Source: CAD feature listing. Evaluate the final solid. Frame: model axes, mm. Face numbers are marked on the shaded views. A direction names the side the tool comes from. Round coordinates to 2 decimals unless told otherwise and drop trailing zeros. Order: outer loops, then holes, each group sorted by start corner. A loop starts at its lowest first (then second) coordinate and runs counter-clockwise, first axis right, second up.
```python
from build123d import *

# Parameters (mm, degrees)
SKETCH1_W           = 6
SKETCH1_H           = 18
BOSS_EXTRUDE1_DEPTH = 2
SKETCH2_R           = 1.5
BOSS_EXTRUDE2_DEPTH = 3
FILLET1_R           = 1.5
SKETCH3_R           = 1.5
SKETCH5_R           = 1
CUT_EXTRUDE1_DEPTH  = 21.686831601


with BuildPart() as part:
    # Sketch1 → Boss-Extrude1 (new body)
    with BuildSketch(Plane.XY):
        Rectangle(SKETCH1_W, SKETCH1_H)
    extrude(amount=BOSS_EXTRUDE1_DEPTH)

    # Sketch2 → Boss-Extrude2 (add)
    with BuildSketch(Plane(origin=(0, 0, 0), x_dir=(-1, 0, 0), z_dir=(0, 0, -1))):
        with Locations((0, 2.35)):
            Circle(SKETCH2_R)
        with Locations((0, -2.62)):
            Circle(SKETCH2_R)
    extrude(amount=BOSS_EXTRUDE2_DEPTH)

    # Fillet1
    fillet1_edges = [part.edges().sort_by_distance(p)[0] for p in [
        (1.5, 2.35, -3),
        (1.5, -2.62, -3),
    ]]
    fillet(fillet1_edges, radius=FILLET1_R)

    # Sweep1: sweep along a path in Sketch4
    with BuildLine(Plane(origin=(0, 2.35, 0), x_dir=(-1, 0, 0), z_dir=(0, 1, 0))) as sweep1_path:
        Line((0, 2), (0, 2.85))
        ThreePointArc((0, 2.85), (-1.757359313, 7.092640687), (-6, 8.85))
        Line((-6, 8.85), (-16.65, 8.85))
    # Sketch3 → Sweep1 (sweep)
    with BuildSketch(Plane.XY.offset(2)):
        with Locations((0, -2.62)):
            Circle(SKETCH3_R)
        with Locations((0, 2.35)):
            Circle(SKETCH3_R)
    sweep(path=sweep1_path.line)

    # Sketch5 → Cut-Extrude1 (cut, through all)
    with BuildSketch(Plane.XY.offset(2)):
        with Locations((0, 6.5)):
            Circle(SKETCH5_R)
        with Locations(Location((0, -6.5, 0), (0, 0, 180))):
            Circle(SKETCH5_R)
    extrude(amount=-CUT_EXTRUDE1_DEPTH, mode=Mode.SUBTRACT)


solid = part.part
```
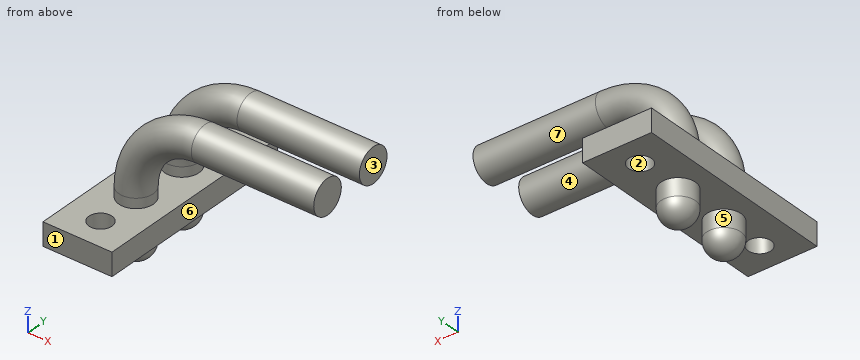
1. Section B-B on z = 2.5. Return loops of the section in (x, y), plus the area to 3 significant figures.
2. Section D-D on y = -2.62. Return loops of the section in (x, z), plus the area to 3 significant figures.
3. Line query: line 1 along Y through (x, z) = (0, 1.55); line 2 along X through (y, z) = (-6.5, 1.25); line 3 along X through (y, z) = (-3.75, 0.75). Output: solid intervals per line, ascending.
4. Access query for the marked faces 5, 6 and 7. Directions: +Z, -Z, +X, -X, +Y, -Y. A direction counts if a zero-diameter tool reaches every point of the face in a straight line with its end or side. Return the directions, or none.
5. Section C-C on x = 9.25. Return loops of the section in (y, z).
6. Pull-direction query (Y, two-part tool) for the marked faces 1, 2, 3 and 4; classes: released by +Y, released by -Y, zero draft, split by the parting line, or undercut.
7. Section A-A on y = -6.5. Return loops of the section in (x, z).
8. First-contact query: pin 1 (2.5 mm diameter, centred on x = 0, y = 6.5, fed in from +Z); pin 2 (10 mm diameter, centred on x = 0, y = 3.5, fed in from +Z); pin 3 (6 mm diameter, centred on x = -0.5, y = -0.5, fed in from +Z). Flat tips, straight axial feed; report the tip coordinate or a pass-through.
Result:
1. outline: circle Ø3 at (0, -2.62); circle Ø3 at (0, 2.35)
1. area: 14.1 mm2
2. outline: (-3, 0) - (-1.5, 0) - (-1.5, -1.5) arc R1.5 ccw to (1.5, -1.5) - (1.5, 0) - (3, 0) - (3, 2) - (1.5, 2) - (1.5, 2.85) arc R4.5 cw to (6, 7.35) - (16.65, 7.35) - (16.65, 10.35) - (6, 10.35) arc R7.5 ccw to (-1.5, 2.85) - (-1.5, 2) - (-3, 2) - close
2. area: 82.8 mm2
3. line 1: y = -9 to -7.5, -5.5 to 5.5, 7.5 to 9
3. line 2: x = -3 to -1, 1 to 3
3. line 3: x = -3 to 3
4. face 5: -Z
4. face 6: -Z, +X, +Y, -Y
4. face 7: +X
5. outline: circle Ø3 at (-2.62, 8.85); circle Ø3 at (2.35, 8.85)
6. face 1: released by -Y
6. face 2: undercut
6. face 3: zero draft
6. face 4: undercut
7. outline: (-3, 0) - (-1, 0) - (-1, 2) - (-3, 2) - close; (1, 0) - (3, 0) - (3, 2) - (1, 2) - close
8. pin 1: stops at z = 2
8. pin 2: stops at z = 10.26
8. pin 3: stops at z = 9.11
